from build123d import *

# Parameters (mm, degrees)
SKETCH1_R      = 10
EXTRUDE1_DEPTH = 5


with BuildPart() as part:
    # Sketch1 → Extrude1 (new body)
    with BuildSketch(Plane.XY):
        Polygon((55, 80), (60, 75), (60, 0), (0, 0), (0, 80), align=None)
        with Locations((30, 40)):
            Circle(SKETCH1_R, mode=Mode.SUBTRACT)
    extrude(amount=-EXTRUDE1_DEPTH)


solid = part.part
Can you work these out from the model? Positions are in its coordinate system, mm. Round coordinates to 2 decimals unless told otherwise and drop trailing zeros. Loops run counter-clockwise (first coordinate to the right, second up) from the corner with the lowest first, then second, coordinate; pieces in that order, holes last. Notation, with made-up numbers: (-6.75, 78) - (46.25, 78) arc R25 cw to (46.25, 112) - close; hole circle Ø8 at (53.5, -1.5). An arc over 180 degrees is marked (long way). Write item = value, one per line. Start each with the question number.
(1) If we section it at B-B (y = 40): Please give me the cut outline in (x, z), and give its area (3 significant figures).
(2) If we mould it in two halves opening along Y, with no side actions, what happens to faces 1 (the face through (27, 80, -2)), 2 (the face through (34.614, 31.128, -2.465)), 3 (the face through (60, 38, -2))? For each: released by +Y, released by -Y, zero draft, split by the parting line, or undercut.
(3) If we section it at C-C (z = -2.6): Please give me the cut outline in (x, y).
(4) If I drill on probe 1 along Y at (x, z) = (30, -2.4); probe 2 along X at (y, z) = (38.5, -4.2); probe 3 along Y at (x, z) = (33.5, -2.6), over which ranges is the centre line in solid material (lowest first)? Write a range as [from, to].
(5) If we section it at A-A (x = 30): Please give me the cut outline in (y, z), and give its area (3 significant figures).
Ans:
q1.outline = (0, -5) - (20, -5) - (20, 0) - (0, 0) - close; (40, -5) - (60, -5) - (60, 0) - (40, 0) - close
q1.area = 200 mm²
q2.face_1 = released by +Y
q2.face_2 = undercut
q2.face_3 = zero draft
q3.outline = (0, 0) - (60, 0) - (60, 75) - (55, 80) - (0, 80) - close; hole circle Ø20 at (30, 40)
q4.probe_1 = [0, 30], [50, 80]
q4.probe_2 = [0, 20.11], [39.89, 60]
q4.probe_3 = [0, 30.63], [49.37, 80]
q5.outline = (0, -5) - (30, -5) - (30, 0) - (0, 0) - close; (50, -5) - (80, -5) - (80, 0) - (50, 0) - close
q5.area = 300 mm²
